Build history of the part. All positions in model axes, mm. Face numbers are marked on the shaded views. A direction names the side the tool comes from. Round coordinates to 2 decimals unless told otherwise and drop trailing zeros. Order: outer loops, then holes, each group sorted by start corner. A loop starts at its lowest first (then second) coordinate and runs counter-clockwise, first axis right, second up. Notation, with made-up numbers: M 3,25 L 50,25 A21 cw 50,59 Z; hole C -7.75,61 d11. An arc over 180 degrees is marked long. Use CSV: the item, a comma, the result in double quotes.
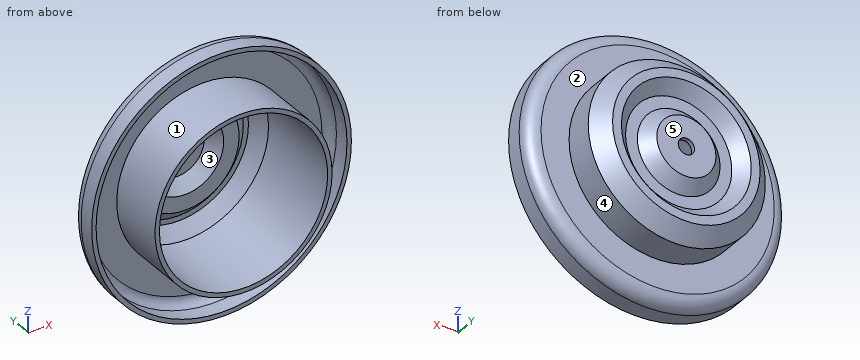
from build123d import *

# Parameters (mm, degrees)
SKETCH_2_R          = 2.75
CUT_EXTRUDE_1_DEPTH = 26
SKETCH_3_R          = 30
SKETCH_3_R_2        = 28.5
EXTRUDE_1_DEPTH     = 20


with BuildPart() as part:
    # Эскиз1 → Повернуть2 (revolve)
    with BuildSketch(Plane.XY):
        with BuildLine():
            Line((0, 0), (10, 0))
            Line((10, 0), (14, -4))
            Line((14, -4), (18, -4))
            Line((18, -4), (22, 0))
            Line((22, 0), (25, 0))
            Line((25, 0), (30, -5))
            Line((30, -5), (30, -15))
            Line((30, -15), (39.5, -15))
            ThreePointArc((39.5, -15), (42.681980515, -16.318019485), (44, -19.5))
            Line((44, -19.5), (44, -25))
            Line((44, -25), (42.5, -25))
            Line((42.5, -25), (42.5, -19.5))
            ThreePointArc((42.5, -19.5), (41.621320344, -17.378679656), (39.5, -16.5))
            Line((39.5, -16.5), (28.5, -16.5))
            Line((28.5, -16.5), (28.5, -5.621320344))
            Line((28.5, -5.621320344), (24.378679656, -1.5))
            Line((24.378679656, -1.5), (22.621320344, -1.5))
            Line((22.621320344, -1.5), (18.621320344, -5.5))
            Line((18.621320344, -5.5), (13.378679656, -5.5))
            Line((13.378679656, -5.5), (9.378679656, -1.5))
            Line((9.378679656, -1.5), (0, -1.5))
            Line((0, -1.5), (0, 0))
        make_face()
    revolve(axis=Axis((0, 0, 0), (0, -1, 0)))

    # Эскиз2 → Вырез-Вытянуть1 (cut, through all)
    with BuildSketch(Plane(origin=(0, 0, 0), x_dir=(1, 0, 0), z_dir=(0, 1, 0))):
        Circle(SKETCH_2_R)
    extrude(amount=-CUT_EXTRUDE_1_DEPTH, mode=Mode.SUBTRACT)

    # Эскиз3 → Бобышка-Вытянуть1 (add)
    with BuildSketch(Plane.XZ.offset(16.5)):
        Circle(SKETCH_3_R)
        Circle(SKETCH_3_R_2, mode=Mode.SUBTRACT)
    extrude(amount=EXTRUDE_1_DEPTH)


solid = part.part
(1) Two-plate mould, pull along X, no slides. Class the marked faces 3, 4 and 5: released by +X, released by -X, zero draft, split by the parting line, or undercut.
Answer block:
face 3,"undercut"
face 4,"split by the parting line"
face 5,"zero draft"
(2) Tool access for the marked faces 1 and 2: list every direction of +Z, -Z, +X, -X, +Y, -Y with a clear straight run to the whole face (end or side of a thin tool).
Answer block:
face 1,"-Y"
face 2,"+Y"
(3) Wall check: line 1 (Z direction, x = 0, y = -21.2); line 2 (Z direction, x = 0, y = -27); line 3 (Z direction, x = 13, y = -19). Give the ranges that are in metal, low to high. Write a range as from..to.
Answer block:
line 1,"z = -44..-42.5, -30..-28.5, 28.5..30, 42.5..44"
line 2,"z = -30..-28.5, 28.5..30"
line 3,"z = -42.01..-40.42, -27.04..-25.36, 25.36..27.04, 40.42..42.01"
(4) Cut at A-A, the plane y = -28. Give the cut face in (x, z), and give its area (3 significant figures).
Answer block:
outline,"C 0,0 d60; hole C 0,0 d57"
area,"276 mm²"
(5) Drop flat-ended pins along their axis: pin 1 (5.5 mm diameter, centred on x = -3.5, z = 3, fed in from -Y); pin 2 (1 mm diameter, centred on x = 11.5, y = -22, fed in from +Z); pin 3 (5 mm diameter, centred on x = -24.5, z = -27, fed in from -Y); pin 4 (4.5 mm diameter, centred on x = 0, z = 0, fed in from +Y). Give the stop position or say it passes through.
Answer block:
pin 1,"stops at y = -1.5"
pin 2,"stops at z = 42.6"
pin 3,"stops at y = -16.5"
pin 4,"passes through"
